Source: CAD feature listing. Evaluate the final solid. Frame: model axes, mm. A direction names the side the tool comes from. Round coordinates to 2 decimals unless told otherwise and drop trailing zeros. Loops run counter-clockwise (first coordinate to the right, second up) from the corner with the lowest first, then second, coordinate; pieces in that order, holes last. Notation, with made-up numbers: (-12, 70.5) - (20, 70.5) arc R8 ccw to (20, 77.5) - close; hole circle Ø8 at (31, 69). An arc over 180 degrees is marked (long way). One line per question, with ' | ' between items. Start each with the question number.
1. Cut plane B-B (x = 33.5). Return loops of the section in (y, z).
2. Pin query (flat end, axial travel): pin 1 (8 mm diameter, centred on x = 10, z = -58.5, fed in from -Y). Return the tip coordinate at first contact, or that it passes through.
3. Cut plane D-D (x = -93.5). Return loops of the section in (y, z), then the cut area to 3 significant figures.
4. Access query for faces 1 (the cylindrical face through (4.88, 37.18, 79.32)), 2 (the flat face through (-152.479, -2, -3)), 3 (the flat face through (-2, 165, 1)). Directions: +Z, -Z, +X, -X, +Y, -Y. A direction counts if a zero-diameter tool reaches every point of the face in a straight line with its end or side. Return the directions, or none.
5. Cut plane A-A (y = 141). Return loops of the section in (x, z).
6. Mould query, pull axis Z, two halves, no side actions, for faces 4 (the flat face through (-2, -2, -83.806)), 5 (the flat face through (151.895, -2, -3)), 6 (the flat face through (141.895, -7, -1)). Classes: pulls with the +Z half, pulls with the -Z half, needs draft (parallel to the pull), parting line crosses it, or undercut.
7. Cut plane C-C (z = 37). Return loops of the section in (x, y).
8. Ray query, line 1 (Z direction, x = 35, y = -44.5); line 2 (X direction, y = 124, z = 53.5); line 3 (Y direction, x = 106, z = -55). Return the intervals inside material, ascending.
```python
from build123d import *

# Parameters (mm, degrees)
F0_W     = 304.373444
F0_H     = 168.19302
F1_DEPTH = 175
F2_T     = -10
F4_D     = 75
F4_DEPTH = 12
F5_R     = 5


with BuildPart() as f1:
    # F0 (on Front) → F1 (new body, symmetric)
    with BuildSketch(Plane.XZ):
        with Locations((-0.291869, 0.29074)):
            Rectangle(F0_W, F0_H)
    extrude(amount=F1_DEPTH, both=True)

    # F2
    f2_openings = [f1.faces().sort_by_distance(p)[0] for p in [
        (-0.291869, -175, 0.29074),
    ]]
    offset(amount=F2_T, openings=f2_openings)

    # F4
    with Locations(Plane.XY.offset(84.38725)):
        with Locations((0, 0)):
            Hole(F4_D / 2, depth=F4_DEPTH)

    # F5
    f5_edges = [f1.edges().sort_by_distance(p)[0] for p in [
        (-152.478591, 0, 84.38725),
        (151.894853, 0, 84.38725),
    ]]
    fillet(f5_edges, radius=F5_R)


solid = f1.part
```
Answers follow:
1) outline: (-175, -83.81) - (175, -83.81) - (175, 84.39) - (16.85, 84.39) - (16.85, 74.39) - (165, 74.39) - (165, -73.81) - (-175, -73.81) - close; (-175, 74.39) - (-16.85, 74.39) - (-16.85, 84.39) - (-175, 84.39) - close
2) pin 1: stops at y = 165
3) outline: (-175, -83.81) - (175, -83.81) - (175, 84.39) - (-175, 84.39) - (-175, 74.39) - (165, 74.39) - (165, -73.81) - (-175, -73.81) - close | area: 8,480 mm2
4) face 1: +Z | face 2: +Z, -Z, -X, +Y, -Y | face 3: -Y
5) outline: (-152.48, -83.81) - (151.89, -83.81) - (151.89, 79.39) arc R5 ccw to (146.89, 84.39) - (-147.48, 84.39) arc R5 ccw to (-152.48, 79.39) - close; hole (-142.48, -73.81) - (141.89, -73.81) - (141.89, 74.39) - (-142.48, 74.39) - close
6) face 4: pulls with the -Z half | face 5: needs draft | face 6: undercut
7) outline: (-152.48, -175) - (-142.48, -175) - (-142.48, 165) - (141.89, 165) - (141.89, -175) - (151.89, -175) - (151.89, 175) - (-152.48, 175) - close
8) line 1: z = -83.81 to -73.81, 74.39 to 84.39 | line 2: x = -152.48 to -142.48, 141.89 to 151.89 | line 3: y = 165 to 175
